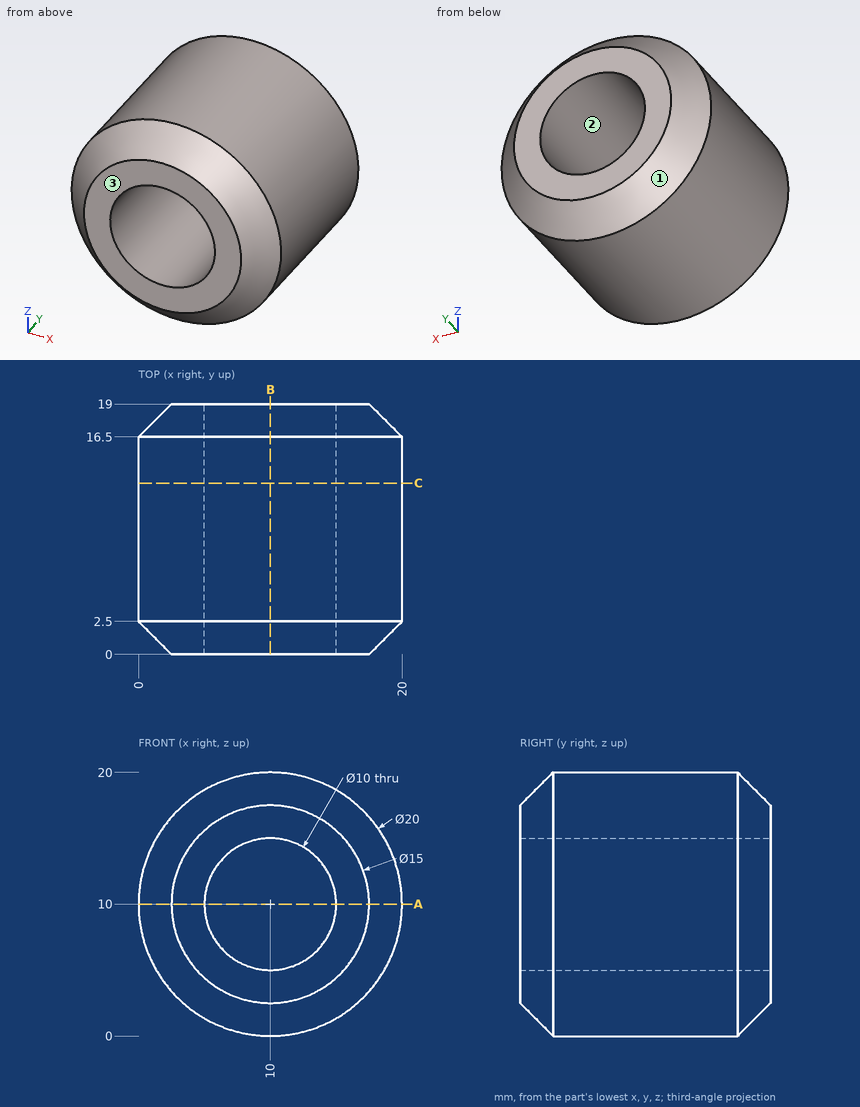
Here's the drawing with two shaded views (mm, measured from the low corner). I have some questions. Give positions to 0.01 mm unless a question says otherwise; leave off trailing zeros. Loops run counter-clockwise (first coordinate to the right, second up) from the corner with the lowest first, then second, coordinate; pieces in that order, holes last. Notation, with made-up numbers: M -14,-12 L 28,-12 A14 cw 28,-8 Z; hole C 54,-4 d10. An arc over 180 degrees is marked long. Use one line per item in the form item = value. Start each with the question number.
Q1. Thinking about a two-plate mould opening in X: for the marked faces 1, 2 and 3, which applies, +X half, -X half, draft (parallel to the pull), parting line (faces both ways), or undercut?
Q2. If we section it at B-B (x = 10): Write out the boundary of the cut face in (y, z).
Q3. If we section it at A-A (z = 10): Write out the boundary of the cut face in (x, y), then the cut area to 4 significant figures.
Q4. I need wall thicknesses on line 1 along X through (y, z) = (15.25, 10); line 2 along Z through (x, y) = (12.75, 10); line 3 along X through (y, z) = (7, 14.25). Which ranges of each line are inside material? Lowest first, please.
Q5. Will these pins go through, and if not, where does the flat tip stop? pin 1 Ø5 at (x, y) = (16.5, 4) entering from -Z; pin 2 Ø10 at (y, z) = (9.5, 2.5) entering from -X; pin 3 Ø8 at (x, z) = (10, 10) entering from -Y; pin 4 Ø5 at (x, y) = (7, 9.5) entering from +Z.
Q6. If we section it at C-C (y = 13): Write out the boundary of the cut face in (x, z).
Taken from the geometry:
q1.face_1 = parting line
q1.face_2 = undercut
q1.face_3 = draft
q2.outline = M 0,2.5 L 2.5,0 L 16.5,0 L 19,2.5 L 19,5 L 0,5 Z; M 0,15 L 19,15 L 19,17.5 L 16.5,20 L 2.5,20 L 0,17.5 Z
q3.outline = M 0,2.5 L 2.5,0 L 5,0 L 5,19 L 2.5,19 L 0,16.5 Z; M 15,0 L 17.5,0 L 20,2.5 L 20,16.5 L 17.5,19 L 15,19 Z
q3.area = 177.5 mm^2
q4.line_1 = 0 to 5, 15 to 20
q4.line_2 = 0.39 to 5.82, 14.18 to 19.61
q4.line_3 = 0.95 to 7.37, 12.63 to 19.05
q5.pin_1 = 0.83
q5.pin_2 = 0.32
q5.pin_3 = through
q5.pin_4 = 19.99
q6.outline = C 10,10 d20; hole C 10,10 d10
